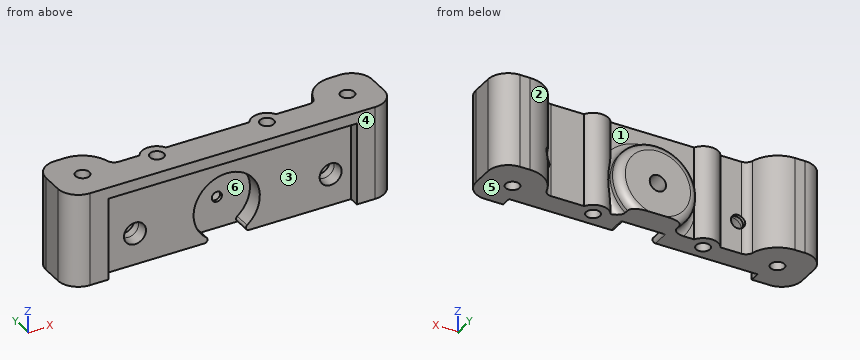
Autodesk Inventor part; units mm, degrees
ref_plane "YZ Plane" through (0, 0, 0) normal (1, 0, 0) x (0, 1, 0)
ref_plane "XZ Plane" through (0, 0, 0) normal (0, 1, 0) x (-1, 0, 0)
ref_plane "XY Plane" through (0, 0, 0) normal (0, 0, 1) x (1, 0, 0)
sketch "Sketch1" plane through (0, 0, 0) normal (0, 0, 1) x (1, 0, 0)
  line L0 (-32.5, 0) -> (32.5, 0) construction
  line L1 (-32.5, -7.5) -> (32.5, -7.5)
  line L2 (32.5, 7.5) -> (-32.5, 7.5)
  arc A0 (-32.5, 7.5) -> (-32.5, -7.5) centre (-32.5, 0) ccw
  arc A1 (32.5, -7.5) -> (32.5, 7.5) centre (32.5, 0) ccw
  arc A2 (-25.0167, 0.5) -> (-32.5, 7.5) centre (-32.5, 0) ccw
  arc A3 (32.5, 7.5) -> (25.0167, 0.5) centre (32.5, 0) ccw
  line L3 (-25.0167, 0.5) -> (25.0167, 0.5)
  point P0 (0, 0)
  point P1 (-32.5, 7.5)
  dimension "d0" = 15
  dimension "d1" = 65
  dimension "d3" = 8
extrude "Extrusion1" add sketch "Sketch1" along normal mid plane 23 contours A0 A2 L3 A3 A1 L1
sketch "Sketch2" plane through (-32.5, 0.5, 11.5) normal (0, -1, 0) x (1, 0, 0)
  line L0 (65, -23) -> (0, -23)
  circle A0 centre (32.5, -15.25) radius 10
  point P0 (32.5, -11.5)
  point P1 (38.8196, -23)
  point P2 (26.1804, -23)
  dimension "d6" = 7.75
  dimension "d14" = 20
extrude "Extrusion2" add sketch "Sketch2" against normal blind 5 contours L0 A0 picked at (30.3633, -19.1493)
sketch "Sketch3" plane through (-32.5, -7.5, 11.5) normal (0, -1, 0) x (1, 0, 0)
  arc A0 (38.8196, -23) -> (26.1804, -23) centre (32.5, -15.25) ccw
  point P0 (32.5, -11.5)
hole "Hole2" at (0, -7.5, -3.75) direction (0, 1, 0) diameter 4 end through all counterbore diameter 16.25 counterbore depth 6.7
fillet "Fillet1" radius 2 4 edges at (0, 0.5, 6.25) (0, 5.5, 6.25) (25.0167, 0.5, 0) (-25.0167, 0.5, 0)
sketch "Sketch5" plane through (-32.5, -7.5, 11.5) normal (0, -1, 0) x (1, 0, 0)
  circle A0 centre (32.5, -15.25) radius 2
  line L0 (63, -2.75) -> (2, -2.75)
  line L1 (2, -2.75) -> (2, -27.75)
  line L2 (2, -27.75) -> (63, -27.75)
  line L3 (63, -27.75) -> (63, -2.75)
  line L4 (63, -2.75) -> (2, -27.75) construction
  line L5 (2, -2.75) -> (63, -27.75) construction
  point P0 (32.5, -11.5)
  dimension "d28" = 61
  dimension "d29" = 12.5
extrude "Extrusion4" cut sketch "Sketch5" against normal blind 2.5
sketch "Sketch6" plane through (0, 0, -11.5) normal (0, 0, -1) x (-1, 0, 0)
  arc A0 (-25.2644, 1.9737) -> (-32.5, -7.5) centre (-32.5, 0) ccw
  arc A1 (32.5, -7.5) -> (25.2644, 1.9737) centre (32.5, 0) ccw
  point P0 (0, 0)
  point P1 (-32.5, 0)
hole "Hole3" at (32.5, 0, -11.5) at (-32.5, 0, -11.5) direction (0, 0, 1) diameter 3.4 end through all
sketch "Sketch7" plane through (0, 0, 11.5) normal (0, 0, 1) x (1, 0, 0)
  circle A0 centre (32.5, 0) radius 1.7
  circle A1 centre (-32.5, 0) radius 1.7
  arc A2 (32.5, -7.5) -> (25.2644, 1.9737) centre (32.5, 0) ccw
  arc A3 (23.3348, 0.5) -> (25.2644, 1.9737) centre (23.3348, 2.5) ccw
  line L0 (23.3348, 0.5) -> (-23.3348, 0.5)
  arc A4 (-25.2644, 1.9737) -> (-23.3348, 0.5) centre (-23.3348, 2.5) ccw
  arc A5 (-25.2644, 1.9737) -> (-32.5, -7.5) centre (-32.5, 0) ccw
  line L1 (-32.5, -7.5) -> (32.5, -7.5)
  arc A6 (-25.2644, 1.9737) -> (-32.5, -7.5) centre (-32.5, 0) ccw
  line L2 (-32.5, 7.5) -> (-35, 7.5)
  line L3 (-40, 2.5) -> (-40, -2.5)
  line L4 (-35, -7.5) -> (-32.5, -7.5)
  arc A7 (-35, 7.5) -> (-40, 2.5) centre (-35, 2.5) ccw
  arc A8 (-40, -2.5) -> (-35, -7.5) centre (-35, -2.5) ccw
  point P0 (0, 0)
  point P1 (-40, 0)
  dimension "d39" = 5
extrude "Extrusion5" add sketch "Sketch7" against normal up to surface (23 mm away) contours L4 A8 L3 A5 | L3 A7 L2 A5
mirror "Mirror1" about plane through (0, 0, 0) normal (1, 0, 0) of "Extrusion5"
sketch "Sketch8" plane through (-32.5, -5, 11.5) normal (0, -1, 0) x (1, 0, 0)
  circle A0 centre (32.5, -15.25) radius 2
  circle A1 centre (58, -15.25) radius 2.65
  circle A2 centre (10, -15.25) radius 2.65
  point P0 (32.5, -11.5)
  dimension "d42" = 25.5
  dimension "d43" = 22.5
  dimension "d44" = 5.3
  dimension "d45" = 5.3
hole "Hole4" at (25.5, -5, -3.75) at (-22.5, -5, -3.75) direction (0, 1, 0) diameter 5 depth 4.75 countersink diameter 5.4 countersink angle 8
sketch "Sketch9" plane through (25.5, -0.25, -3.75) normal (0, -1, 0) x (1, 0, 0)
  circle A0 centre (0, 0) radius 2.7
  circle A1 centre (-48, 0) radius 2.5
  point P0 (-25.5, 3.75)
hole "Hole5" at (25.5, -0.25, -3.75) at (-22.5, -0.25, -3.75) direction (0, 1, 0) diameter 3.4 depth 9.5
sketch "Sketch11" plane through (0, 0, -11.5) normal (0, 0, -1) x (-1, 0, 0)
  circle A0 centre (-12, -1.3) radius 2.7
  circle A1 centre (15, -1.3) radius 2.7
  line L0 (-30.5, -5) -> (-2.4399, -5)
  circle A2 centre (-12, -1.3) radius 3.7
  circle A3 centre (15, -1.3) radius 3.7
  line L1 (30.5, -7.5) -> (-30.5, -7.5)
  point P0 (0, 0)
  dimension "d71" = 5.4
  dimension "d72" = 5.4
  dimension "d73" = 15
  dimension "d74" = 12
  dimension "d76" = 1
  dimension "d94" = 6.2
extrude "Extrusion6" add sketch "Sketch11" against normal up to surface (23 mm away) contours A0 | A1 | A2 | A3
sketch "Sketch12" plane through (0, 0, -11.5) normal (0, 0, -1) x (-1, 0, 0)
  arc A0 (-8.7792, 0.5211) -> (-15.2326, 0.5) centre (-12, -1.3) ccw
  arc A1 (18.2326, 0.5) -> (11.7674, 0.5) centre (15, -1.3) ccw
  point P0 (0, 0)
  point P1 (-13.7674, 0.5)
hole "Hole7" at (12, -1.3, -11.5) at (-15, -1.3, -11.5) direction (0, 0, 1) diameter 3.4 end through all
fillet "Fillet2" radius 0.75 2 edges at (2.4399, -2.9, -11.5) (-2.4399, -2.9, -11.5)
sketch "Sketch15" plane through (0, -0.8, -3.75) normal (0, -1, 0) x (1, 0, 0)
  circle A0 centre (0, 0) radius 2
  circle A1 centre (0, 0) radius 1.25
  point P0 (0, 3.75)
  dimension "d103" = 0.75
extrude "Extrusion7" add sketch "Sketch15" against normal blind 0.75
properties part number "Lower Extruder Block" material "ABS Plastic"
For this review, take the finished solid that the model builds, in its own axes (mm). Face numbers are marked on the shaded views. A direction names the side the tool comes from. Coordinates: 2 decimals unless noted, no trailing zeros. Loops run counter-clockwise (first coordinate to the right, second up) from the corner with the lowest first, then second, coordinate; pieces in that order, holes last. Notation, with made-up numbers: (3, 22) - (51, 22) arc R30 cw to (51, 53) - close; hole circle Ø10 at (1, 50). An arc over 180 degrees is marked (long way). Use a Markdown table: item, result. Add a question column.
Item 1: Insertion check: pin 1 Ø2 at (y, z) = (-6, -4) entering from -X; pin 2 Ø10 at (x, z) = (-18.5, 3) entering from -Y; pin 3 Ø2.5 at (x, z) = (-22, -3) entering from +Y. Each pin has a flat end and moves straight along its axis. Give the tip position at first contact, or say it passes through.
Item 2: We need section D-D (x = 0). Give the boundary of the cut face in (y, z) (3 decimals).
Item 3: For line 1 (X direction, y = -2, z = 1.5); line 2 (X direction, y = 3.6, z = -3.75); line 3 (X direction, y = 3, z = 2.25), list the stretches that pass through material, from the lowest coordinate up.
Item 4: We need section A-A (x = -22.5). Give the boundary of the cut face in (y, z), and give its area (3 significant figures).
Item 5: We need section B-B (y = 6.25). Give the boundary of the cut face in (x, z), and give its area (3 significant figures).
Item 6: We need section C-C (z = -3.75). Give the number of separate pieces and of enclosed holes in the cut face, and give its area (3 significant figures).
Item 7: Tool access review of the marked faces 1, 2 and 3: name each direction out of +Z, -Z, +X, -X, +Y, -Y from which nothing blocks a thin tool from reaching the whole face with its end or side.
Item 8: Mouldability with a two-part tool opening along Z and no side actions: class the marked faces 4, 5 and 6 as pulls with the +Z half, pulls with the -Z half, needs draft (parallel to the pull), parting line crosses it, or undercut.
Results list:
| question | item | result |
|---|---|---|
| 1 | pin 1 | stops at x = -39.33 |
| 1 | pin 2 | stops at y = -5 |
| 1 | pin 3 | stops at y = 0.5 |
| 2 | outline | (-7.5, 8.75) - (-5, 8.75) - (-5, 4.375) - (-0.8, 4.375) - (-0.8, -2.5) - (-0.05, -2.5) - (-0.05, -1.75) - (5.5, -1.75) - (5.5, 4.25) arc R2 ccw to (3.5, 6.25) - (2.5, 6.25) arc R2 cw to (0.5, 8.25) - (0.5, 11.5) - (-7.5, 11.5) - close; (-0.8, -11.5) - (5.5, -11.5) - (5.5, -5.75) - (-0.05, -5.75) - (-0.05, -5) - (-0.8, -5) - close |
| 3 | line 1 | x = -40 to -16.55, -13.45 to -6.2, 6.2 to 10.45, 13.55 to 40 |
| 3 | line 2 | x = -39.88 to -25.92, -10 to -2, 2 to 10, 27.2 to 39.88 |
| 3 | line 3 | x = -39.97 to -25.63, -8 to 8, 25.63 to 39.97 |
| 4 | outline | (-7.5, 8.75) - (-5, 8.75) - (-5, -1.05) - (-2.14, -1.25) - (-0.25, -1.25) - (-0.25, -2.05) - (0.5, -2.05) - (0.5, 11.5) - (-7.5, 11.5) - close; (-5, -11.5) - (0.5, -11.5) - (0.5, -5.45) - (-0.25, -5.45) - (-0.25, -6.25) - (-2.14, -6.25) - (-5, -6.45) - close |
| 4 | area | 107 mm^2 |
| 5 | outline | (-38.31, -11.5) - (-28.35, -11.5) - (-28.35, 11.5) - (-38.31, 11.5) - close; (28.35, -11.5) - (38.31, -11.5) - (38.31, 11.5) - (28.35, 11.5) - close |
| 5 | area | 458 mm^2 |
| 6 | separate pieces | 4 |
| 6 | enclosed holes | 4 |
| 6 | area | 579 mm^2 |
| 7 | face 1 | +Z, +Y |
| 7 | face 2 | +Z, -Z, +Y |
| 7 | face 3 | -Z, -Y |
| 8 | face 4 | needs draft |
| 8 | face 5 | pulls with the -Z half |
| 8 | face 6 | undercut |
